Can you work these out from the model? Positions are in its coordinate system, mm. A direction names the side the tool comes from. Coordinates: 2 decimals unless noted, no trailing zeros. Order: outer loops, then holes, each group sorted by start corner. A loop starts at its lowest first (then second) coordinate and runs counter-clockwise, first axis right, second up. Notation, with made-up numbers: (40, 18.5) -> (93, 18.5) arc R17 ccw to (93, 44.5) -> close; hole circle Ø2 at (77.25, 58.5). An arc over 180 degrees is marked (long way). Use a Markdown table: item, result. Add a question column.
1. For faces 1 (the flat face through (3, -1.5, 0)), 2 (the flat face through (3, 1.5, 0)), which set-ups out of +Z, -Z, +X, -X, +Y, -Y let a thin tool reach every point of the face, with its end or its side?
2. For pin 1 Ø3 at (x, z) = (302, -2.5) entering from +Y; pin 2 Ø1.1 at (y, z) = (2.5, -1) entering from -X; pin 3 Ø5 at (x, z) = (32.5, -3.5) entering from -Y, each with a flat end and sliding along its axis, tell me the tip position at first contact or that it passes through.
3. If I drill on line 1 along X through (y, z) = (0.5, 2.25); line 2 along X through (y, z) = (0.5, -2); line 3 along X through (y, z) = (1.75, -1), over which ranges is the centre line in solid material (lowest first)? Write a range as from..to.
4. Suppose I cut it at B-B, the plane x = 0. List the corners of the cut face in (y, z) for me, then the cut area to 3 significant figures.
5. Suppose I cut it at A-A, the plane x = 300. List the corners of the cut face in (y, z) for me, then the cut area to 3 significant figures.
6. Suppose I cut it at C-C, the plane x = 216.5. List the corners of the cut face in (y, z) for me.
7. We'd pull the mould along X, two halves only. Please class faces 3 (the cylindrical face through (152, -3, 0)), 4 (the cylindrical face through (-5, 0, 0)), 5 (the flat face through (302.5, 1.5, 1.2)): pulls with the +X half, pulls with the -X half, needs draft (parallel to the pull), parting line crosses it, or undercut.
```python
from build123d import *

# Parameters (mm, degrees)
F1_R         = 5
F1_R_2       = 2
F2_DEPTH     = 1.5
F5_R         = 3
F6_DEPTH     = 146
F9_T4_ANGLE  = 354.9348896549
F9_T9_ANGLE  = 354.9348896549
F9_S10_R     = 3
F9_T11_DEPTH = 9
F9_T15_ANGLE = 354.9348896549
F9_T20_ANGLE = 354.9348896549
F9_S21_R     = 3
F9_T22_DEPTH = 9


# Not quite as in the source:
# - a fillet or chamfer that OpenCascade refuses, or shapes differently, is made with other operations: its cross-section is extruded or revolved along the edge and cut away or added


with BuildPart() as f2:
    # F1 (on Front) → F2 (new body, symmetric)
    with BuildSketch(Plane.XZ):
        Circle(F1_R)
        Circle(F1_R_2, mode=Mode.SUBTRACT)
    extrude(amount=F2_DEPTH, both=True)

    # F0 (on Top) → F3 (revolve, cut)
    with BuildSketch(Plane.XY):
        with BuildLine():
            Line((1.5, 2.5980762114), (1.5, -2.5980762114))
            ThreePointArc((1.5, -2.5980762114), (3, 0), (1.5, 2.5980762114))
        make_face()
    revolve(axis=Axis((0, 0.5133161101, 0), (0, -1, 0)), mode=Mode.SUBTRACT)

    # F5 (on offset) → F6 (join)
    with BuildSketch(Plane.YZ.offset(4)):
        Circle(F5_R)
    extrude(amount=F6_DEPTH)

    # F8: F2 across plane


with BuildPart() as f2_1:
    add(f2.part)
    add(f2.part.mirror(Plane.YZ.offset(150)))

    # F9: fillet of radius 1 on 2 edges, made by hand


with BuildPart() as f9_tool2:
    # F9_s3 → F9_t4 (revolve)
    with BuildSketch(Plane(origin=(0, 0, 0), x_dir=(0, 1, 0), z_dir=(0.0441870344, 0, -0.999023276))):
        with BuildLine():
            ThreePointArc((-0.5, 5), (-1.2071067812, 4.7071067812), (-1.5, 4))
            Line((-1.5, 4), (-1.5, 5))
            Line((-1.5, 5), (-0.5, 5))
        make_face()
    revolve(axis=Axis((0, -1.5, 0), (0, -1, 0)), revolution_arc=F9_T4_ANGLE)

    split(bisect_by=Plane.YZ.offset(4), keep=Keep.BOTTOM)


with BuildPart() as f2_2:
    add(f2_1.part)

    # F9_t1: cut F9_tool2
    add(f9_tool2.part, mode=Mode.SUBTRACT)


with BuildPart() as f9_tool7:
    # F9_s8 → F9_t9 (revolve)
    with BuildSketch(Plane(origin=(0, 0, 0), x_dir=(0, 1, 0), z_dir=(0.0441870344, 0, -0.999023276))):
        with BuildLine():
            ThreePointArc((-0.5, 5), (-1.2071067812, 4.7071067812), (-1.5, 4))
            Line((-1.5, 4), (-1.5, 5))
            Line((-1.5, 5), (-0.5, 5))
        make_face()
    revolve(axis=Axis((0, -1.5, 0), (0, -1, 0)), revolution_arc=F9_T9_ANGLE)

    # F9_s10 → F9_t11 (cut, symmetric)
    with BuildSketch(Plane.YZ):
        Circle(F9_S10_R)
    extrude(amount=F9_T11_DEPTH, both=True, mode=Mode.SUBTRACT)


with BuildPart() as f2_3:
    add(f2_2.part)

    # F9_t6: cut F9_tool7
    add(f9_tool7.part, mode=Mode.SUBTRACT)


with BuildPart() as f9_tool13:
    # F9_s14 → F9_t15 (revolve)
    with BuildSketch(Plane(origin=(0, 0, 0), x_dir=(0, 1, 0), z_dir=(0.0441870344, 0, -0.999023276))):
        with BuildLine():
            ThreePointArc((0.5, 5), (1.2071067812, 4.7071067812), (1.5, 4))
            Line((1.5, 4), (1.5, 5))
            Line((1.5, 5), (0.5, 5))
        make_face()
    revolve(axis=Axis((0, 1.5, 0), (0, -1, 0)), revolution_arc=F9_T15_ANGLE)

    split(bisect_by=Plane.YZ.offset(4), keep=Keep.BOTTOM)


with BuildPart() as f2_4:
    add(f2_3.part)

    # F9_t12: cut F9_tool13
    add(f9_tool13.part, mode=Mode.SUBTRACT)


with BuildPart() as f9_tool18:
    # F9_s19 → F9_t20 (revolve)
    with BuildSketch(Plane(origin=(0, 0, 0), x_dir=(0, 1, 0), z_dir=(0.0441870344, 0, -0.999023276))):
        with BuildLine():
            ThreePointArc((0.5, 5), (1.2071067812, 4.7071067812), (1.5, 4))
            Line((1.5, 4), (1.5, 5))
            Line((1.5, 5), (0.5, 5))
        make_face()
    revolve(axis=Axis((0, 1.5, 0), (0, -1, 0)), revolution_arc=F9_T20_ANGLE)

    # F9_s21 → F9_t22 (cut, symmetric)
    with BuildSketch(Plane.YZ):
        Circle(F9_S21_R)
    extrude(amount=F9_T22_DEPTH, both=True, mode=Mode.SUBTRACT)


with BuildPart() as f2_5:
    add(f2_4.part)

    # F9_t17: cut F9_tool18
    add(f9_tool18.part, mode=Mode.SUBTRACT)


solid = f2_5.part
```
Worked out:
| question | item | result |
|---|---|---|
| 1 | face 1 | +Z, -Z, -X, -Y |
| 1 | face 2 | +Z, -Z, -X, +Y |
| 2 | pin 1 | stops at y = 1.5 |
| 2 | pin 2 | stops at x = 4 |
| 2 | pin 3 | stops at y = -2.83 |
| 3 | line 1 | x = -4.47..-1.92, 1.92..298.08, 301.92..304.47 |
| 3 | line 2 | x = -4.58..-2.18, 2.18..297.82, 302.18..304.58 |
| 3 | line 3 | x = 4..296 |
| 4 | outline | (-1.5, -4) arc R1 ccw to (-0.5, -5) -> (0.5, -5) arc R1 ccw to (1.5, -4) -> (1.5, -2.6) arc R3 cw to (-1.5, -2.6) -> close; (-1.5, 2.6) arc R3 cw to (1.5, 2.6) -> (1.5, 4) arc R1 ccw to (0.5, 5) -> (-0.5, 5) arc R1 ccw to (-1.5, 4) -> close |
| 4 | area | 11.9 mm² |
| 5 | outline | (-1.5, -5) -> (1.5, -5) -> (1.5, -2.6) arc R3 cw to (-1.5, -2.6) -> close; (-1.5, 2.6) arc R3 cw to (1.5, 2.6) -> (1.5, 5) -> (-1.5, 5) -> close |
| 5 | area | 12.8 mm² |
| 6 | outline | circle Ø6 at (0, 0) |
| 7 | face 3 | undercut |
| 7 | face 4 | undercut |
| 7 | face 5 | needs draft |
